from build123d import *

# Parameters (mm, degrees)
BOSS_EXTRUDE2_DEPTH = 10
SKETCH2_R           = 2.5
BOSS_EXTRUDE3_DEPTH = 20
SKETCH4_R           = 2.5
CUT_EXTRUDE1_DEPTH  = 41
FILLET1_R           = 1.25


with BuildPart() as part:
    # Sketch1 → Boss-Extrude2 (new body)
    with BuildSketch(Plane.XY):
        with BuildLine():
            Line((-80, 5), (-30, 5))
            ThreePointArc((-30, 5), (-16.666666667, 10.09288015), (-10.1238402, 22.777777778))
            ThreePointArc((-10.1238402, 22.777777778), (-9.305986892, 24.363389981), (-7.639320225, 25))
            Line((-7.639320225, 25), (-5, 25))
            Line((-5, 25), (-5, 15))
            Line((-5, 15), (5, 15))
            Line((5, 15), (5, -15))
            Line((5, -15), (-5, -15))
            Line((-5, -15), (-5, -25))
            Line((-5, -25), (-7.639320225, -25))
            ThreePointArc((-7.639320225, -25), (-9.305986892, -24.363389981), (-10.1238402, -22.777777778))
            ThreePointArc((-10.1238402, -22.777777778), (-16.666666667, -10.09288015), (-30, -5))
            Line((-30, -5), (-80, -5))
            Line((-80, -5), (-80, 5))
        make_face()
    extrude(amount=BOSS_EXTRUDE2_DEPTH)

    # Sketch2 → Boss-Extrude3 (add)
    with BuildSketch(Plane.ZY.offset(80)):
        with Locations((5, 0)):
            Circle(SKETCH2_R)
    extrude(amount=BOSS_EXTRUDE3_DEPTH)

    # Sketch3 → Revolve1 (revolve)
    with BuildSketch(Plane.ZY.offset(100)):
        with BuildLine():
            Line((5, 10), (5, -10))
            ThreePointArc((5, -10), (-5, 0), (5, 10))
        make_face()
    revolve(axis=Axis((-100, 10, 5), (0, -1, 0)))

    # Sketch4 → Cut-Extrude1 (cut, through all)
    with BuildSketch(Plane(origin=(0, 15, 0), x_dir=(1, 0, 0), z_dir=(0, 1, 0))):
        with Locations((0, -5)):
            Circle(SKETCH4_R)
    extrude(amount=-CUT_EXTRUDE1_DEPTH, mode=Mode.SUBTRACT)

    # Fillet1
    fillet1_edges = [part.edges().sort_by_distance(p)[0] for p in [
        (-16.666666667, -10.09288015, 10),
        (-55, 5, 0),
        (-16.666666667, 10.09288015, 0),
        (-9.305986892, 24.363389981, 0),
        (-6.319660113, 25, 0),
        (-5, 20, 0),
        (0, 15, 0),
        (5, 0, 0),
        (0, -15, 0),
        (-9.305986892, -24.363389981, 10),
        (-5, -20, 0),
        (-6.319660113, -25, 0),
        (-9.305986892, -24.363389981, 0),
        (-16.666666667, -10.09288015, 0),
        (-55, -5, 0),
        (-80, 0, 0),
        (-6.319660113, -25, 10),
        (-80, 5, 5),
        (-5, 25, 5),
        (5, 15, 5),
        (5, -15, 5),
        (-5, -25, 5),
        (-5, -20, 10),
        (-80, -5, 5),
        (0, -15, 10),
        (5, 0, 10),
        (0, 15, 10),
        (-5, 20, 10),
        (-6.319660113, 25, 10),
        (-9.305986892, 24.363389981, 10),
        (-80, 0, 10),
        (-16.666666667, 10.09288015, 10),
        (-55, 5, 10),
        (-55, -5, 10),
    ]]
    fillet(fillet1_edges, radius=FILLET1_R)


solid = part.part
Source: CAD feature listing. Evaluate the final solid. Frame: model axes, mm. A direction names the side the tool comes from. Coordinates: 2 decimals unless noted, no trailing zeros. Loops run counter-clockwise (first coordinate to the right, second up) from the corner with the lowest first, then second, coordinate; pieces in that order, holes last. Notation, with made-up numbers: (-11.75, 22) - (27.25, 22) arc R18 cw to (27.25, 51) - close; hole circle Ø8 at (9.25, -26). An arc over 180 degrees is marked (long way). One line per item, written item: value. Start each with the question number.
1. Section B-B (z = 5). Return the cut outline in (x, y).
2. Set-up query: faces 4 (the cylindrical face through (-16.515, -10.23, 4.948)), 5 (the flat face through (-55, 5, 5)), 6 (the flat face through (-25, 0, 10)), 7 (the cylindrical face through (-85.087, 0.751, 7.385)), 8 (the flat face through (-5, -19, 5)). Return all of +Z, -Z, +X, -X, +Y, -Y with unobstructed straight access to the full face (end or side cutting, diameter ignored); none if empty.
3. Section C-C (y = 0). Return the cut outline in (x, z), and give its area (3 significant figures).
4. Section A-A (x = 0). Return the cut outline in (y, z).
5. Section D-D (x = -38.5). Return the cut outline in (y, z).
6. Contact query for flat-ended pins moving along their axis: P1, Ø1, axis at x = -98.5, y = -12, coming from the +Z side; P2, Ø6.5, axis at x = 0, z = 5, coming from the +Y side; P3, Ø6, axis at y = 1, z = 6.5, coming from the -X side; P4, Ø4, axis at y = 17.5, z = 3.5, coming from the +X side. Output: stop coordinate, or through.
7. Mould query, pull axis X, two halves, no side actions, for faces 1 (the flat face through (-25, 0, 0)), 2 (the cylindrical face through (-0.33, 0.21, 2.52)), 3 (the flat face through (-5, 19, 5)). Classes: pulls with the +X half, pulls with the -X half, needs draft (parallel to the pull), parting line crosses it, or undercut.
8. Ray query, L1, parallel to Z at x = 0, y = -5.75; L2, parallel to X at y = 0, z = 5; L3, parallel to X at y = 8.5, z = 5. Return the intervals inside material, ascending.
Verdict:
1. outline: (-90.32, -2.5) - (-80, -2.5) - (-80, -3.75) arc R1.25 ccw to (-78.75, -5) - (-30, -5) arc R20 cw to (-10.12, -22.78) arc R2.5 ccw to (-7.64, -25) - (-6.25, -25) arc R1.25 ccw to (-5, -23.75) - (-5, -15) - (-2.5, -15) - (-2.5, 15) - (-5, 15) - (-5, 23.75) arc R1.25 ccw to (-6.25, 25) - (-7.64, 25) arc R2.5 ccw to (-10.12, 22.78) arc R20 cw to (-30, 5) - (-78.75, 5) arc R1.25 ccw to (-80, 3.75) - (-80, 2.5) - (-90.32, 2.5) arc R10 ccw (long way) to start; (2.5, -15) - (3.75, -15) arc R1.25 ccw to (5, -13.75) - (5, 13.75) arc R1.25 ccw to (3.75, 15) - (2.5, 15) - close
2. face 4: +Z, -Z, -Y
2. face 5: +Z, -Z, +Y
2. face 6: +Z, +X, +Y, -Y
2. face 7: none
2. face 8: +Z, -Z, +X, -Y
3. outline: (-90.32, 2.5) - (-80, 2.5) - (-80, 1.25) arc R1.25 ccw to (-78.75, 0) - (3.75, 0) arc R1.25 ccw to (5, 1.25) - (5, 8.75) arc R1.25 ccw to (3.75, 10) - (-78.75, 10) arc R1.25 ccw to (-80, 8.75) - (-80, 7.5) - (-90.32, 7.5) arc R10 ccw (long way) to start; hole circle Ø5 at (0, 5)
3. area: 1,190 mm2
4. outline: (-15, 1.25) arc R1.25 ccw to (-13.75, 0) - (13.75, 0) arc R1.25 ccw to (15, 1.25) - (15, 2.5) - (-15, 2.5) - close; (-15, 7.5) - (15, 7.5) - (15, 8.75) arc R1.25 ccw to (13.75, 10) - (-13.75, 10) arc R1.25 ccw to (-15, 8.75) - close
5. outline: (-5, 1.25) arc R1.25 ccw to (-3.75, 0) - (3.75, 0) arc R1.25 ccw to (5, 1.25) - (5, 8.75) arc R1.25 ccw to (3.75, 10) - (-3.75, 10) arc R1.25 ccw to (-5, 8.75) - close
6. P1: passes through
6. P2: stops at y = 15
6. P3: stops at x = -110
6. P4: stops at x = -5
7. face 1: needs draft
7. face 2: undercut
7. face 3: pulls with the +X half
8. L1: z = 0 to 2.5, 7.5 to 10
8. L2: x = -110 to -2.5, 2.5 to 5
8. L3: x = -105.27 to -94.73, -18.7 to -2.5, 2.5 to 5
